Autodesk Inventor part; units mm, degrees
ref_plane "YZ Plane" through (0, 0, 0) normal (1, 0, 0) x (0, 1, 0)
ref_plane "XZ Plane" through (0, 0, 0) normal (0, 1, 0) x (-1, 0, 0)
ref_plane "XY Plane" through (0, 0, 0) normal (0, 0, 1) x (1, 0, 0)
sketch "Sketch1" plane through (0, 0, 0) normal (0, 1, 0) x (-1, 0, 0)
  circle A0 centre (0, 0) radius 6
  dimension "d3" = 12
extrude "Extrusion1" add sketch "Sketch1" along normal mid plane 12
sketch "Sketch2" plane through (0, 6, 0) normal (0, 1, 0) x (1, 0, 0)
  line L0 (1.5326, 3.1066) -> (3.4567, 0.226)
  line L1 (3.4567, 0.226) -> (1.9241, -2.8806)
  line L2 (1.9241, -2.8806) -> (-1.5326, -3.1066)
  line L3 (-1.5326, -3.1066) -> (-3.4567, -0.226)
  line L4 (-3.4567, -0.226) -> (-1.9241, 2.8806)
  line L5 (-1.9241, 2.8806) -> (1.5326, 3.1066)
  point P0 (0, 0)
  point P1 (0, 0)
  dimension "d2" = 6
extrude "Extrusion2" cut sketch "Sketch2" against normal blind 5.5
thread "Thread1"
chamfer "Chamfer1" distance 0.5 angle 45 2 edges at (6, 6, 0) (6, -6, 0)
properties part number "M12_HEX"
Model file for the job. Use its own axes, mm. A direction names the side the tool comes from. Give positions to 0.01 mm unless a question says otherwise; leave off trailing zeros. Order: outer loops, then holes, each group sorted by start corner. A loop starts at its lowest first (then second) coordinate and runs counter-clockwise, first axis right, second up.
1) Saw through at B-B, the plane x = 0. Write the cut outline in (y, z), then the cut area to 3 significant figures.
2) Saw through at D-D, the plane y = -4.5. Write the cut outline in (x, z), then the cut area to 3 significant figures.
3) 3-axis set-ups, long thin cutter, end or side, ignore diameter. For faces 1 (the flat face through (-0.22, 3.288, -2.992)), 2 (the flat face through (-2.4, 6, -2.4)): which of +Z, -Z, +X, -X, +Y, -Y reach the whole face in a straight line?
4) Saw through at A-A, the plane y = 4. Write the cut outline in (x, z), then the cut area to 3 significant figures.
5) Saw through at C-C, the plane z = 0. Write the cut outline in (x, y).
6) Wall check: probe 1 along Y at (x, z) = (-0.5, 0.75); probe 2 along Z at (x, y) = (-3, 2); probe 3 along X at (y, z) = (1.5, -1.25). Give the ranges that are in metal, low to high.
7) Mould opens along X. For faces 3 (the flat face through (0, -6, 0)), 4 (the flat face through (0, 0.5, 0)), 5 (the cylindrical face through (6, 0, 0)) say: +X half, -X half, draft (parallel to the pull), parting line (faces both ways), or undercut.
8) Pin check, flat tips, straight feed: pin 1 (5 mm diameter, centred on x = 4.5, y = -4.5, fed in from -Z); pin 2 (1.5 mm diameter, centred on y = 2, z = -3.5, fed in from -X). Stop position of each tip, or through.
Computed:
1. outline: (-6, -5.5) - (-5.5, -6) - (5.5, -6) - (6, -5.5) - (6, -3.01) - (0.5, -3.01) - (0.5, 3.01) - (6, 3.01) - (6, 5.5) - (5.5, 6) - (-5.5, 6) - (-6, 5.5) - close
1. area: 110 mm2
2. outline: circle Ø12 at (0, 0)
2. area: 113 mm2
3. face 1: +Y
3. face 2: +Z, -Z, +X, -X, +Y
4. outline: circle Ø12 at (0, 0); hole (-3.46, 0.23) - (-1.92, -2.88) - (1.53, -3.11) - (3.46, -0.23) - (1.92, 2.88) - (-1.53, 3.11) - close
4. area: 81.9 mm2
5. outline: (-6, -5.5) - (-5.5, -6) - (5.5, -6) - (6, -5.5) - (6, 5.5) - (5.5, 6) - (3.35, 6) - (3.35, 0.5) - (-3.35, 0.5) - (-3.35, 6) - (-5.5, 6) - (-6, 5.5) - close
6. probe 1: y = -6 to 0.5
6. probe 2: z = -5.2 to -0.7, 0.91 to 5.2
6. probe 3: x = -5.87 to -2.73, 2.77 to 5.87
7. face 3: draft
7. face 4: undercut
7. face 5: parting line
8. pin 1: stops at z = -5.66
8. pin 2: stops at x = -5.33
